The listing builds one solid part. Answer for the finished solid, in the listing's coordinates (mm). A direction names the side the tool comes from. Round coordinates to 2 decimals unless told otherwise and drop trailing zeros. Order: outer loops, then holes, each group sorted by start corner. A loop starts at its lowest first (then second) coordinate and runs counter-clockwise, first axis right, second up. Notation, with made-up numbers: (64, -32.75) -> (77, -32.75) arc R26 ccw to (77, -0.75) -> close; hole circle Ø5 at (22, 51). An arc over 180 degrees is marked (long way). Answer in a Markdown table with one row per item. Add a question column.
```python
from build123d import *

# Parameters (mm, degrees)
F0_R     = 2
F0_W     = 16
F0_H     = 12.7209685743
F0_W_2   = 10
F0_H_2   = 5
F1_DEPTH = 6
F3_W     = 10
F3_H     = 1.5
F4_DEPTH = 25
F5_W     = 11
F5_H     = 6
F5_W_2   = 10
F5_H_2   = 5
F6_DEPTH = 4


with BuildPart() as f1:
    # F0 (on Front) → F1 (new body)
    with BuildSketch(Plane.XZ):
        with BuildLine():
            ThreePointArc((-4, 23), (-4.1246826636, 24.216818062), (-4.493548732, 25.383064085))
            ThreePointArc((-4.493548732, 25.383064085), (-10, 29), (-15.506451268, 25.383064085))
            ThreePointArc((-15.506451268, 25.383064085), (-11.216818062, 17.1246826636), (-4, 23))
        make_face()
        with Locations((-10, 23)):
            Circle(F0_R, mode=Mode.SUBTRACT)
        with BuildLine():
            Line((-20, 15), (0, 15))
            Line((0, 15), (-4.493548732, 25.383064085))
            ThreePointArc((-4.493548732, 25.383064085), (-4.1246826636, 24.216818062), (-4, 23))
            ThreePointArc((-4, 23), (-11.216818062, 17.1246826636), (-15.506451268, 25.383064085))
            Line((-15.506451268, 25.383064085), (-20, 15))
        make_face()
        Polygon((-2, 0), (0, 0), (0, 15), (-20, 15), (-20, 0), (-18, 0), (-18, 12.7209685743), (-2, 12.7209685743), align=None)
        with Locations((-10, 6.3604842871)):
            Rectangle(F0_W, F0_H)
        with Locations((-10, 7.5)):
            Rectangle(F0_W_2, F0_H_2, mode=Mode.SUBTRACT)
        with Locations((-10, 7.5)):
            Rectangle(F0_W_2, F0_H_2)
    extrude(amount=F1_DEPTH)

    # F3 (on line) → F4 (cut)
    with BuildSketch(Plane(origin=(0, 0, 12.7209685743), x_dir=(1, 0, 0), z_dir=(0, 0, -1))):
        with Locations((-10, 2.75)):
            Rectangle(F3_W, F3_H)
    extrude(amount=F4_DEPTH, mode=Mode.SUBTRACT)

    # F5 (on face) → F6 (cut)
    with BuildSketch(Plane.XZ.offset(6)):
        with Locations((-10, 7.5)):
            Rectangle(F5_W, F5_H)
        with Locations((-10, 7.5)):
            Rectangle(F5_W_2, F5_H_2, mode=Mode.SUBTRACT)
        with Locations((-10, 7.5)):
            Rectangle(F5_W_2, F5_H_2)
    extrude(amount=-F6_DEPTH, mode=Mode.SUBTRACT)


solid = f1.part
```
Item 1: Flat-ended cylindrical pins translate along their axes: P1, Ø1, axis at x = -13.5, y = -2, coming from the +Z side; P2, Ø2, axis at x = -12.5, y = -4, coming from the +Z side; P3, Ø1, axis at y = -3.5, z = 20, coming from the +X side. Find the tip coordinate at first contact, or state that the pin passes through.
Item 2: Find the intervals of material crossed by probe 1 along Z at (x, y) = (-10, -4.7); probe 2 along X at (y, z) = (-5.2, 10); probe 3 along Z at (x, y) = (-10, -1.45), in increasing order. Write a range as [from, to].
Item 3: The part is cut by section D-D, the plane z = 24. Give the vertices of the cut face in (x, y) (3 decimals).
Item 4: For a pull along Y with two mould halves and no side action, classify faces 1 (the face through (-10, 0, 11)), 2 (the face through (-10, -2, 6)), 3 (the face through (0, -3, 7)) as released by +Y, released by -Y, zero draft, split by the parting line, or undercut.
Item 5: The part is cut by section C-C, the plane x = -10. Give the vertices of the cut face in (y, z).
Item 6: The part is cut by section A-A, the plane y = -0.5. Give the vertices of the cut face in (x, z), and give its area (3 significant figures).
Item 7: The part is cut by section B-B, the plane z = 7.75. Give the vertices of the cut face in (x, y).
Item 8: A tool of negligible diameter and unlimited length cuts with its end or side. For faces 4 (the face through (-15.5, -4, 7)), 5 (the face through (-17.722, -2.958, 20.264)), 6 (the face through (-5, -3, 12)), from which of +Z, -Z, +X, -X, +Y, -Y can it reach the whole face along a straight path? Write none if from no direction.
Resolved:
| question | item | result |
|---|---|---|
| 1 | P1 | z = 28.2 |
| 1 | P2 | z = 28.81 |
| 1 | P3 | x = -1.95 |
| 2 | probe 1 | [0, 4.5], [10.5, 21], [25, 29] |
| 2 | probe 2 | [-20, -15.5], [-4.5, 0] |
| 2 | probe 3 | [0, 21], [25, 29] |
| 3 | outline | (-16.105, -6) -> (-11.732, -6) -> (-11.732, 0) -> (-16.105, 0) -> close; (-8.268, -6) -> (-3.895, -6) -> (-3.895, 0) -> (-8.268, 0) -> close |
| 4 | face 1 | released by +Y |
| 4 | face 2 | undercut |
| 4 | face 3 | zero draft |
| 5 | outline | (-6, 0) -> (-3.5, 0) -> (-3.5, 4.5) -> (-6, 4.5) -> close; (-6, 10.5) -> (-3.5, 10.5) -> (-3.5, 12.72) -> (-2, 12.72) -> (-2, 0) -> (0, 0) -> (0, 21) -> (-6, 21) -> close; (-6, 25) -> (0, 25) -> (0, 29) -> (-6, 29) -> close |
| 6 | outline | (-20, 0) -> (0, 0) -> (0, 15) -> (-4.49, 25.38) arc R6 ccw to (-15.51, 25.38) -> (-20, 15) -> close; hole circle Ø4 at (-10, 23) |
| 6 | area | 477 mm2 |
| 7 | outline | (-20, -6) -> (-15.5, -6) -> (-15.5, -2) -> (-4.5, -2) -> (-4.5, -6) -> (0, -6) -> (0, 0) -> (-20, 0) -> close |
| 8 | face 4 | -Y |
| 8 | face 5 | +Z, -X, +Y, -Y |
| 8 | face 6 | -Z |
